from build123d import *

# Parameters (mm, degrees)
SKETCH2_R           = 4.7625
BOSS_EXTRUDE1_DEPTH = 3.175


with BuildPart() as part:
    # Sketch1 → Revolve1 (revolve)
    with BuildSketch(Plane.XY, mode=Mode.PRIVATE) as revolve1_sk:
        Polygon((0, 0), (1.9812, 0), (1.9812, 25.4), (3.175, 25.4), (3.175, 55.626), (1.6637, 55.626), (1.6637, 61.087), (0, 61.087), align=None)
    revolve(revolve1_sk.sketch.rotate(Axis((0, 0, 0), (0, 1, 0)), 90), axis=Axis((0, 0, 0), (0, 1, 0)))  # turned: the seam where the file's is

    # Sketch2 → Boss-Extrude1 (add)
    with BuildSketch(Plane.XZ.offset(-25.4)):
        with Locations(Location((0, 0, 0), (0, 0, 270))):  # turned: the seam where the file's is
            Circle(SKETCH2_R)
    extrude(amount=-BOSS_EXTRUDE1_DEPTH)


solid = part.part
Design review of the part built by this model. Coordinates are the model's own, in mm. A direction names the side the tool comes from. Round coordinates to 2 decimals unless told otherwise and drop trailing zeros. Loops run counter-clockwise (first coordinate to the right, second up) from the corner with the lowest first, then second, coordinate; pieces in that order, holes last. Notation, with made-up numbers: M 14.5,73 L 54.5,73 A27 cw 54.5,111 Z; hole C 13,-9 d6. An arc over 180 degrees is marked long. Answer as a JSON object with one key per item and string values.
Item 1: Clearance check with flat-ended pins moving along their axes: P1, Ø1.5, axis at y = 37, z = 2.5, coming from the +X side; P2, Ø5, axis at y = 27, z = -3, coming from the -X side; P3, Ø1, axis at x = -2.5, y = 37.5, coming from the +Z side. State where each tip first meets the part, or that it passes through.
Answer sheet:
{"P1": "stops at x = 2.65", "P2": "stops at x = -4.74", "P3": "stops at z = 2.47"}
Item 2: Wall thickness on L1, parallel to Y at x = 1, z = -3.75 (3 decimals); L2, parallel to X at y = 34, z = 0.25; L3, parallel to Y at x = -1.25, z = -2.5: over which ranges is each line inside the solid? List them lowest first. Write a range as from..to.
Answer sheet:
{"L1": "y = 25.4..28.575", "L2": "x = -3.17..3.17", "L3": "y = 25.4..55.63"}
Item 3: We need section D-D on y = 27. Give the boundary of the cut face in (x, z) (1 decimal).
Answer sheet:
{"outline": "C 0,0 d9.5"}
Item 4: Machinability: for faces 1 (the flat face through (0, 0, 0)), 2 (the flat face through (-2, 25.4, -1)), 3 (the flat face through (1.4, 55.626, -1.4)), which of the approach directions +Z, -Z, +X, -X, +Y, -Y give a long, thin tool a straight path to every point of the face, cutting with its end or side? Answer none if there is none.
Answer sheet:
{"face 1": "+Z, -Z, +X, -X, -Y", "face 2": "-Y", "face 3": "+Y"}
Item 5: We need section B-B on z = 0. Give the boundary of the cut face in (x, y) (1 decimal), and give its area (3 significant figures).
Answer sheet:
{"outline": "M -4.8,25.4 L -2,25.4 L -2,0 L 2,0 L 2,25.4 L 4.8,25.4 L 4.8,28.6 L 3.2,28.6 L 3.2,55.6 L 1.7,55.6 L 1.7,61.1 L -1.7,61.1 L -1.7,55.6 L -3.2,55.6 L -3.2,28.6 L -4.8,28.6 Z", "area": "321 mm^2"}
Item 6: We need section C-C on y = 40.5. Give the boundary of the cut face in (x, z) (3 decimals), and give its area (3 significant figures).
Answer sheet:
{"outline": "C 0,0 d6.35", "area": "31.7 mm^2"}
Item 7: We need section A-A on x = 0. Give the boundary of the cut face in (y, z) (1 decimal), and give its area (3 significant figures).
Answer sheet:
{"outline": "M 0,-2 L 25.4,-2 L 25.4,-4.8 L 28.6,-4.8 L 28.6,-3.2 L 55.6,-3.2 L 55.6,-1.7 L 61.1,-1.7 L 61.1,1.7 L 55.6,1.7 L 55.6,3.2 L 28.6,3.2 L 28.6,4.8 L 25.4,4.8 L 25.4,2 L 0,2 Z", "area": "321 mm^2"}
